Design review of the part built by this model. Coordinates are the model's own, in mm. A direction names the side the tool comes from. Coordinates: 2 decimals unless noted, no trailing zeros. One line per question, with ' | ' between items.
from build123d import *

# Parameters (mm, degrees)
F0_W     = 1.444232
F0_H     = 3.282842
F0_W_2   = 1.444231
F0_H_2   = 3.003372
F0_W_3   = 1.537525
F0_W_4   = 1.486413
F0_H_3   = 3.08099
F0_H_4   = 3.080991
F1_DEPTH = 25.4


with BuildPart() as f1:
    # F0 (on Top) → F1 (new body)
    with BuildSketch(Plane.XY):
        Polygon((-48.942287, 71.072713), (-59.440054, 71.072713), (-59.440054, 0), (-57.754032, 0), (-55.809505, 0), (-52.57833, 0), (-50.541282, 0), (-48.942287, 0), align=None)
        with Locations((-56.983804, 2.812295)):
            Rectangle(F0_W, F0_H, mode=Mode.SUBTRACT)
        with Locations((-56.872925, 7.838232)):
            Rectangle(F0_W, F0_H, mode=Mode.SUBTRACT)
        with Locations((-56.872925, 16.510591)):
            Rectangle(F0_W, F0_H, mode=Mode.SUBTRACT)
        Polygon((-57.521909, 24.464175), (-57.521909, 24.561059), (-56.077678, 24.561059), (-56.077678, 24.464175), (-56.077678, 21.557687), (-57.521909, 21.557687), align=None, mode=Mode.SUBTRACT)
        with Locations((-56.799793, 28.910887)):
            Rectangle(F0_W_2, F0_H_2, mode=Mode.SUBTRACT)
        with Locations((-56.799793, 35.114071)):
            Rectangle(F0_W_2, F0_H_2, mode=Mode.SUBTRACT)
        with Locations((-52.395074, 2.811296)):
            Rectangle(F0_W, F0_H, mode=Mode.SUBTRACT)
        with Locations((-52.558644, 7.978718)):
            Rectangle(F0_W, F0_H, mode=Mode.SUBTRACT)
        with Locations((-52.576316, 16.499392)):
            Rectangle(F0_W_2, F0_H_2, mode=Mode.SUBTRACT)
        with Locations((-52.70471, 23.120777)):
            Rectangle(F0_W_3, F0_H_2, mode=Mode.SUBTRACT)
        with Locations((-52.988848, 28.910887)):
            Rectangle(F0_W, F0_H_2, mode=Mode.SUBTRACT)
        with Locations((-53.189216, 35.114071)):
            Rectangle(F0_W, F0_H_2, mode=Mode.SUBTRACT)
        with Locations((-57.582847, 40.996084)):
            Rectangle(F0_W_4, F0_H_3, mode=Mode.SUBTRACT)
        with Locations((-57.582847, 46.210064)):
            Rectangle(F0_W_4, F0_H_3, mode=Mode.SUBTRACT)
        with Locations((-56.933529, 50.743902)):
            Rectangle(F0_W_4, F0_H_3, mode=Mode.SUBTRACT)
        with Locations((-56.628476, 55.987162)):
            Rectangle(F0_W_4, F0_H_4, mode=Mode.SUBTRACT)
        with Locations((-56.686215, 61.655125)):
            Rectangle(F0_W_4, F0_H_3, mode=Mode.SUBTRACT)
        with Locations((-56.646839, 67.83214)):
            Rectangle(F0_W_4, F0_H_3, mode=Mode.SUBTRACT)
        with Locations((-53.198363, 40.344337)):
            Rectangle(F0_W_4, F0_H_3, mode=Mode.SUBTRACT)
        with Locations((-52.879221, 50.743902)):
            Rectangle(F0_W_4, F0_H_3, mode=Mode.SUBTRACT)
        with Locations((-52.724365, 45.499066)):
            Rectangle(F0_W_4, F0_H_3, mode=Mode.SUBTRACT)
        with Locations((-52.879221, 56.218265)):
            Rectangle(F0_W_4, F0_H_3, mode=Mode.SUBTRACT)
        with Locations((-52.871432, 61.655125)):
            Rectangle(F0_W_4, F0_H_3, mode=Mode.SUBTRACT)
        with Locations((-52.871499, 67.4915)):
            Rectangle(F0_W_4, F0_H_3, mode=Mode.SUBTRACT)
    extrude(amount=F1_DEPTH)


solid = f1.part
1. Tool access review of faces 1 (the face through (-59.44, 36, 13)), 2 (the face through (-58, 44.67, 13)): name each direction out of +Z, -Z, +X, -X, +Y, -Y from which nothing blocks a thin tool from reaching the whole face with its end or side.
Answer sheet:
face 1: +Z, -Z, -X, +Y, -Y | face 2: +Z, -Z
2. Take a section at A-A (z = 12.75). Count the separate pieces of the cut face and the enclosed holes in it, then the cut area to 3 significant figures.
Answer sheet:
separate pieces: 1 | enclosed holes: 24 | area: 637 mm^2
3. Insertion check: pin 1 Ø1.2 at (x, z) = (-57.5, 16) entering from -Y. The pin has a flat end and moves straight along its axis. Give the tip position at first contact, or say it passes through.
Answer sheet:
pin 1: y = 0
4. To check wall thickness, follow line 1 along X through (y, z) = (51.5, 6.75); line 2 along X through (y, z) = (62, 18); line 3 along X through (y, z) = (42.5, 14.25). State the ranges of each line that lie inside material, in increasing order. Write a range as [from, to].
Answer sheet:
line 1: [-59.44, -57.68], [-56.19, -53.62], [-52.14, -48.94] | line 2: [-59.44, -57.43], [-55.94, -53.61], [-52.13, -48.94] | line 3: [-59.44, -58.33], [-56.84, -48.94]
5. Draft analysis for pull direction Y (two halves, no side actions). For faces 3 (the face through (-52.467, 35, 13)), 4 (the face through (-54.3, 36, 0)), state which applies: pulls with the +Y half, pulls with the -Y half, needs draft (parallel to the pull), parting line crosses it, or undercut.
Answer sheet:
face 3: undercut | face 4: needs draft
